Geometry check sheet. Reference: the model listing, model coordinates, mm. Round coordinates to 2 decimals unless told otherwise and drop trailing zeros. Use one line per item in the form item = value.
from build123d import *

# Parameters (mm, degrees)
SZKIC1_W                    = 63.27
SZKIC1_H                    = 168
DODANIE_WYCI_GNI_CIE1_DEPTH = 6
SZKIC5_R                    = 1.55
WYTNIJ_WYCI_GNI_CIE1_DEPTH  = 6
SZYK_LINIOWY1_COUNT         = 2
SZYK_LINIOWY1_PITCH         = 16


with BuildPart() as part:
    # Szkic1 → Dodanie-wyciągnięcie1 (new body)
    with BuildSketch(Plane.XY):
        with Locations((1183.133039301, -877.922207314)):
            Rectangle(SZKIC1_W, SZKIC1_H)
    extrude(amount=DODANIE_WYCI_GNI_CIE1_DEPTH)

    # Szkic5 → Wytnij-wyciągnięcie1 (cut)
    with BuildSketch(Plane.XY.offset(6)):
        with Locations((1203.133039301, -956.822207314)):
            Circle(SZKIC5_R)
        with Locations((1163.133039301, -956.822207314)):
            Circle(SZKIC5_R)
        with Locations((1163.133039301, -886.922207314)):
            Circle(SZKIC5_R)
        with Locations((1203.133039301, -886.922207314)):
            Circle(SZKIC5_R)
        with Locations((1203.133039301, -801.922207314)):
            Circle(SZKIC5_R)
        with Locations((1163.133039301, -801.922207314)):
            Circle(SZKIC5_R)
    wytnij_wyci_gni_cie1 = extrude(amount=-WYTNIJ_WYCI_GNI_CIE1_DEPTH, mode=Mode.SUBTRACT)

    # Szyk liniowy1: Wytnij-wyciągnięcie1 ×2
    with Locations(*[(0, -i * SZYK_LINIOWY1_PITCH, 0) for i in range(1, SZYK_LINIOWY1_COUNT)]):
        add(wytnij_wyci_gni_cie1, mode=Mode.SUBTRACT)


solid = part.part
1. Mould release check, pull along X, two halves, no side actions. Record for faces 1 (the cylindrical face through (1201.991, -901.875, 3.042)), 2 (the cylindrical face through (1201.991, -816.875, 3.042)), 3 (the flat face through (1183, -793.922, 3)), 4 (the flat face through (1214.768, -879, 3)): released by +X, released by -X, zero draft, split by the parting line, or undercut.
Return value:
face_1 = undercut
face_2 = undercut
face_3 = zero draft
face_4 = released by +X
2. Gauge pin test, flat end, axial feed: pin 1 (2.5 mm diameter, centred on x = 1163.13, y = -902.92, fed in from +Z). Record the tip position at first contact, or that the pin passes through.
Return value:
pin_1 = through
3. Material ranges on line 1 along X through (y, z) = (-904, 2.7); line 2 along Y through (x, z) = (1162, 0.75), recorded low to high.
Return value:
line_1 = 1151.5 to 1162.02, 1164.25 to 1202.02, 1204.25 to 1214.77
line_2 = -961.92 to -957.88, -955.76 to -903.98, -901.86 to -887.98, -885.86 to -818.98, -816.86 to -802.98, -800.86 to -793.92
